```python
from build123d import *

# Parameters (mm, degrees)
SKETCH1_W           = 19.9
SKETCH1_H           = 10.25
BOSS_EXTRUDE1_DEPTH = 6.15
SKETCH2_W           = 12
SKETCH2_H           = 1
CUT_EXTRUDE1_DEPTH  = 6.15
FILLET1_SIZE        = 1
FILLET2_R           = 0.35
SKETCH3_W           = 2
SKETCH3_H           = 3
BOSS_EXTRUDE2_DEPTH = 1.7
CUT_EXTRUDE2_DEPTH  = 21.5
SKETCH5_R           = 1.25
CUT_EXTRUDE3_DEPTH  = 21.5
SKETCH6_W           = 2.5
SKETCH6_H           = 0.8
BOSS_EXTRUDE3_DEPTH = 6.15
FILLET3_R           = 0.1
SKETCH7_W           = 0.5
SKETCH7_H           = 3.35
BOSS_EXTRUDE4_DEPTH = 4
SKETCH8_R           = 0.675
CUT_EXTRUDE4_DEPTH  = 44
FILLET4_R           = 0.35
BOSS_EXTRUDE5_START = -1.1
SKETCH9_W           = 0.4
SKETCH9_H           = 1
BOSS_EXTRUDE5_DEPTH = 4
CUT_EXTRUDE7_DEPTH  = 24
FILLET6_R           = 0.35


with BuildPart() as part:
    # Sketch1 → Boss-Extrude1 (new body)
    with BuildSketch(Plane.XY):
        with Locations((9.95, 5.125)):
            Rectangle(SKETCH1_W, SKETCH1_H)
    extrude(amount=BOSS_EXTRUDE1_DEPTH)

    # Sketch2 → Cut-Extrude1 (cut)
    with BuildSketch(Plane.XY.offset(6.15)):
        with Locations((13.9, 9.75)):
            Rectangle(SKETCH2_W, SKETCH2_H)
    extrude(amount=-CUT_EXTRUDE1_DEPTH, mode=Mode.SUBTRACT)

    # Fillet1
    fillet1_edges = [part.edges().sort_by_distance(p)[0] for p in [
        (7.9, 9.25, 3.075),
    ]]
    chamfer(fillet1_edges, length=FILLET1_SIZE - 0.0001)  # a hair under: the kernel refuses the full size

    # Fillet2
    fillet2_edges = [part.edges().sort_by_distance(p)[0] for p in [
        (19.9, 9.25, 3.075),
        (0, 10.25, 3.075),
        (19.9, 0, 3.075),
        (0, 0, 3.075),
    ]]
    fillet(fillet2_edges, radius=FILLET2_R)

    # Sketch3 → Boss-Extrude2 (add)
    with BuildSketch(Plane(origin=(0, 10.25, 0), x_dir=(1, 0, 0), z_dir=(0, 1, 0))):
        with Locations((6.5, -3.072396368)):
            Rectangle(SKETCH3_W, SKETCH3_H)
    extrude(amount=BOSS_EXTRUDE2_DEPTH)

    # Sketch4 → Cut-Extrude2 (cut)
    with BuildSketch(Plane.XY.offset(4.572396368)):
        with BuildLine():
            Line((5.5, 11.95), (5.5, 11.55))
            ThreePointArc((5.5, 11.55), (5.961483519, 11.846291202), (6.5, 11.95))
            Line((6.5, 11.95), (5.5, 11.95))
        make_face()
        with BuildLine():
            Line((7.5, 11.95), (6.5, 11.95))
            ThreePointArc((6.5, 11.95), (7.038516481, 11.846291202), (7.5, 11.55))
            Line((7.5, 11.55), (7.5, 11.95))
        make_face()
    extrude(amount=-CUT_EXTRUDE2_DEPTH, mode=Mode.SUBTRACT)

    # Sketch5 → Cut-Extrude3 (cut)
    with BuildSketch(Plane.XY.offset(6.15)):
        with Locations((5.05, 2.55)):
            Circle(SKETCH5_R)
        with Locations((14.65, 2.55)):
            Circle(SKETCH5_R)
    extrude(amount=-CUT_EXTRUDE3_DEPTH, mode=Mode.SUBTRACT)

    # Sketch6 → Boss-Extrude3 (add)
    with BuildSketch(Plane.XY.offset(6.15)):
        with Locations((5.05, -0.4)):
            Rectangle(SKETCH6_W, SKETCH6_H)
        with Locations((14.65, -0.4)):
            Rectangle(SKETCH6_W, SKETCH6_H)
    extrude(amount=-BOSS_EXTRUDE3_DEPTH)

    # Fillet3
    fillet3_edges = [part.edges().sort_by_distance(p)[0] for p in [
        (15.9, -0.8, 3.075),
        (13.4, -0.8, 3.075),
        (6.3, -0.8, 3.075),
        (3.8, -0.8, 3.075),
    ]]
    fillet(fillet3_edges, radius=FILLET3_R)

    # Sketch7 → Boss-Extrude4 (add)
    with BuildSketch(Plane.XZ):
        with Locations((2.075, 3.075)):
            Rectangle(SKETCH7_W, SKETCH7_H)
        with Locations((17.825, 3.075)):
            Rectangle(SKETCH7_W, SKETCH7_H)
        with Locations((9.95, 3.075)):
            Rectangle(SKETCH7_W, SKETCH7_H)
    extrude(amount=BOSS_EXTRUDE4_DEPTH)

    # Sketch8 → Cut-Extrude4 (cut)
    with BuildSketch(Plane.ZY.offset(-1.825)):
        with Locations((3.075, -2.5)):
            Circle(SKETCH8_R)
    extrude(amount=-CUT_EXTRUDE4_DEPTH, mode=Mode.SUBTRACT)

    # Fillet4
    fillet4_edges = [part.edges().sort_by_distance(p)[0] for p in [
        (2.075, -4, 1.4),
        (2.075, -4, 4.75),
        (17.825, -4, 4.75),
        (17.825, -4, 1.4),
        (9.95, -4, 4.75),
        (9.95, -4, 1.4),
    ]]
    fillet(fillet4_edges, radius=FILLET4_R)

    # Sketch9 → Boss-Extrude5 (add)
    with BuildSketch(Plane.XY.offset(6.15).offset(BOSS_EXTRUDE5_START)):
        with Locations((2.65, 10.75)):
            Rectangle(SKETCH9_W, SKETCH9_H)
        with BuildLine():
            Line((2.392566175, 11.441575979), (19.634404289, 16.61062023))
            ThreePointArc((19.634404289, 16.61062023), (19.883414093, 16.476478076), (19.749271939, 16.227468271))
            Line((19.749271939, 16.227468271), (2.507433825, 11.058424021))
            ThreePointArc((2.507433825, 11.058424021), (2.258424021, 11.192566175), (2.392566175, 11.441575979))
        make_face()
    extrude(amount=-BOSS_EXTRUDE5_DEPTH)

    # Sketch12 → Cut-Extrude7 (cut)
    with BuildSketch(Plane.XY.offset(5.05)):
        with BuildLine():
            Line((2.392566175, 11.441575979), (2.692202246, 11.531405851))
            add(Edge.make_bspline(
                [(2.45, 11.05), (2.461499925, 11.421364666), (2.692202246, 11.531405851)],
                knots=[0, 0, 0, 0.800009839, 0.800009839, 0.800009839], degree=2))
            ThreePointArc((2.45, 11.05), (2.252117212, 11.220975836), (2.392566175, 11.441575979))
        make_face()
    extrude(amount=-CUT_EXTRUDE7_DEPTH, mode=Mode.SUBTRACT)

    # Fillet6
    fillet6_edges = [part.edges().sort_by_distance(p)[0] for p in [
        (2.85, 11.161124192, 3.05),
    ]]
    fillet(fillet6_edges, radius=FILLET6_R)


solid = part.part
```
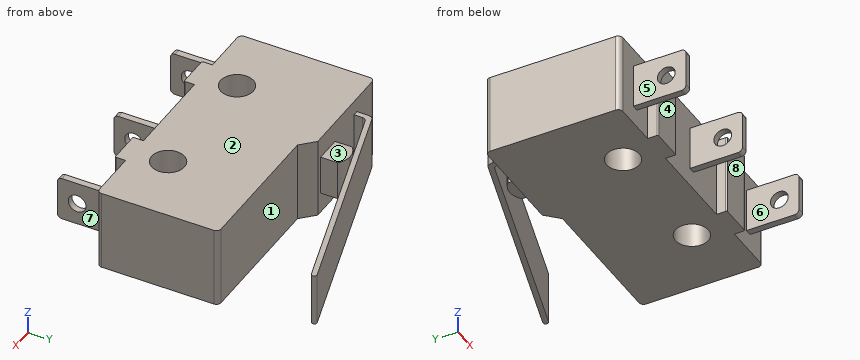
Geometry: final body of the model. Coordinates: model frame, mm. Face numbers are marked on the shaded views. A direction names the side the tool comes from. Give positions to 0.01 mm unless a question says otherwise; leave off trailing zeros. Write each loop counter-clockwise with the first axis right and the second up, starting at its lowest first coordinate (ties: lowest second). Pieces come first, ordered by that corner, then holes.
1. Pin query (flat end, axial travel): P1, Ø1, axis at y = 11, z = 2.5, coming from the +X side; P2, Ø3, axis at x = 8, z = 4, coming from the -Y side; P3, Ø5, axis at x = 13.5, y = 12, coming from the -Z side; P4, Ø1.9, axis at x = 11.5, y = 12.5, coming from the +Z side. Return the tip coordinate at first contact, or that it passes through.
2. Reachability of the marked faces 1, 2, 3 and 4 from +Z, -Z, +X, -X, +Y, -Y: full face, straight path, thin tool, end or side. Return the list, or none.
3. Line query: probe 1 along X at (y, z) = (2.5, 3); probe 2 along Y at (x, z) = (14.65, 4); probe 3 along X at (y, z) = (3.25, 1). Output: solid intervals per line, ascending.
4. Section query D-D, the plane y = -2.5. Return loops of the section in (x, z) (3 decimals).
5. Section query B-B, the plane z = 5.5. Count the separate pieces of the cut face and the enclosed holes in it, then the cut area to 3 significant figures.
6. Section query C-C, the plane x = 14.65. Return loops of the section in (y, z), then the cut area to 3 significant figures.
7. Draft query along X for the marked faces 5, 6, 7 and 8. Return one class per face: released by +X, released by -X, zero draft, split by the parting line, or undercut.
8. Section query A-A, the plane y = 2.55. Return loops of the section in (x, z), then the cut area to 3 significant figures.
Computed:
1. P1: stops at x = 7.5
1. P2: stops at y = 0
1. P3: stops at z = 1.05
1. P4: passes through
2. face 1: +Z, -Z, +X
2. face 2: +Z, +X, -X, +Y, -Y
2. face 3: +Z, +X
2. face 4: +Z, -Z, -Y
3. probe 1: x = 0 to 3.8, 6.3 to 13.4, 15.9 to 19.9
3. probe 2: y = -0.8 to 1.3, 3.8 to 9.25, 14.7 to 15.12
3. probe 3: x = 0 to 4.01, 6.09 to 13.61, 15.69 to 19.9
4. outline: (1.825, 1.4) - (2.325, 1.4) - (2.325, 2.4) - (1.825, 2.4) - close; (1.825, 3.75) - (2.325, 3.75) - (2.325, 4.75) - (1.825, 4.75) - close; (9.7, 1.4) - (10.2, 1.4) - (10.2, 2.4) - (9.7, 2.4) - close; (9.7, 3.75) - (10.2, 3.75) - (10.2, 4.75) - (9.7, 4.75) - close; (17.575, 1.4) - (18.075, 1.4) - (18.075, 2.4) - (17.575, 2.4) - close; (17.575, 3.75) - (18.075, 3.75) - (18.075, 4.75) - (17.575, 4.75) - close
5. separate pieces: 1
5. enclosed holes: 2
5. area: 187 mm2
6. outline: (-0.8, 0) - (1.3, 0) - (1.3, 6.15) - (-0.8, 6.15) - close; (3.8, 0) - (9.25, 0) - (9.25, 6.15) - (3.8, 6.15) - close; (14.7, 1.05) - (15.12, 1.05) - (15.12, 5.05) - (14.7, 5.05) - close
6. area: 48.1 mm2
7. face 5: released by -X
7. face 6: undercut
7. face 7: released by +X
7. face 8: undercut
8. outline: (0, 0) - (3.8, 0) - (3.8, 6.15) - (0, 6.15) - close; (6.3, 0) - (13.4, 0) - (13.4, 6.15) - (6.3, 6.15) - close; (15.9, 0) - (19.9, 0) - (19.9, 6.15) - (15.9, 6.15) - close
8. area: 91.6 mm2
